Could you check a few things on this model? Use its own coordinates, in mm. A direction names the side the tool comes from. Round coordinates to 2 decimals unless told otherwise and drop trailing zeros. Write each loop counter-clockwise with the first axis right and the second up, starting at its lowest first coordinate (ties: lowest second). Pieces come first, ordered by that corner, then holes. Notation, with made-up numbers: (7, 86) -> (11, 86) arc R23 ccw to (11, 124) -> close; hole circle Ø8 at (46, 72.5). An arc over 180 degrees is marked (long way). Answer in a Markdown table with one row per item. Add a question column.
```python
from build123d import *

# Parameters (mm, degrees)
F0_W     = 800
F0_H     = 510
F1_DEPTH = 18
F2_W     = 18
F2_H     = 510
F3_DEPTH = 750
F4_W     = 18
F4_H     = 510
F5_DEPTH = 750
F6_W     = 510
F6_H     = 18
F7_DEPTH = 764


with BuildPart() as f1:
    # F0 (on Top) → F1 (new body)
    with BuildSketch(Plane.XY):
        Rectangle(F0_W, F0_H)
    extrude(amount=F1_DEPTH)

    # F2 (on face) → F3 (join)
    with BuildSketch(Plane.XY.offset(18)):
        with Locations((-391, 0)):
            Rectangle(F2_W, F2_H)
    extrude(amount=F3_DEPTH)

    # F4 (on face) → F5 (join)
    with BuildSketch(Plane.XY.offset(18)):
        with Locations((391, 0)):
            Rectangle(F4_W, F4_H)
    extrude(amount=F5_DEPTH)

    # F6 (on face) → F7 (join)
    with BuildSketch(Plane(origin=(382, 0, 0), x_dir=(0, -1, 0), z_dir=(-1, 0, 0))):
        with Locations((0, 759)):
            Rectangle(F6_W, F6_H)
    extrude(amount=F7_DEPTH)


solid = f1.part
```
(1) If we mould it in two halves opening along Z, with no side actions, what happens to faces 3 (the face through (-6, 4, 0)), 4 (the face through (-382, -4, 379)), 5 (the face through (6, 4, 768))? For each: pulls with the +Z half, pulls with the -Z half, needs draft (parallel to the pull), parting line crosses it, or undercut.
(2) Suppose I cut it at B-B, the plane x = -54. Please give me the cut outline in (y, z).
(3) For P1, Ø5, axis at x = 104.5, y = -177, coming from the -Z side, with a flat end and sliding along its axis, tell me the tip position at first contact or that it passes through.
(4) Suppose I cut it at C-C, the plane y = 133. Please give me the cut outline in (x, z), then the cut area to 3 significant figures.
(5) On a 3-axis mill with a long thin cutter (end or side, diameter ignored), from which of +Z, -Z, +X, -X, +Y, -Y can I reach the whole of each face in a straight line? I mean faces 1 (the face through (382, -4, 379)), 2 (the face through (-400, -4, 379)). Say none if no direction works.
(6) Suppose I cut it at A-A, the plane z = 552.5. Please give me the cut outline in (x, y).
(7) I need wall thicknesses on L1, parallel to Z at x = -276.5, y = -25; L2, parallel to X at y = 121, z = 254.5. Which ranges of each line are inside material? Lowest first, please.
Response:
| question | item | result |
|---|---|---|
| 1 | face 3 | pulls with the -Z half |
| 1 | face 4 | undercut |
| 1 | face 5 | pulls with the +Z half |
| 2 | outline | (-255, 0) -> (255, 0) -> (255, 18) -> (-255, 18) -> close; (-255, 750) -> (255, 750) -> (255, 768) -> (-255, 768) -> close |
| 3 | P1 | z = 0 |
| 4 | outline | (-400, 0) -> (400, 0) -> (400, 768) -> (-400, 768) -> close; hole (-382, 18) -> (382, 18) -> (382, 750) -> (-382, 750) -> close |
| 4 | area | 55,200 mm² |
| 5 | face 1 | +Y, -Y |
| 5 | face 2 | +Z, -Z, -X, +Y, -Y |
| 6 | outline | (-400, -255) -> (-382, -255) -> (-382, 255) -> (-400, 255) -> close; (382, -255) -> (400, -255) -> (400, 255) -> (382, 255) -> close |
| 7 | L1 | 0 to 18, 750 to 768 |
| 7 | L2 | -400 to -382, 382 to 400 |
